Autodesk Inventor part; units mm, degrees
ref_plane "YZ Plane" through (0, 0, 0) normal (1, 0, 0) x (0, 1, 0)
ref_plane "XZ Plane" through (0, 0, 0) normal (0, 1, 0) x (-1, 0, 0)
ref_plane "XY Plane" through (0, 0, 0) normal (0, 0, 1) x (1, 0, 0)
sketch "Sketch1" plane through (0, 0, 0) normal (0, 1, 0) x (-1, 0, 0)
  line L0 (44.45, 203.2) -> (-44.45, 203.2)
  line L1 (-44.45, 203.2) -> (-44.45, -203.2)
  line L2 (-44.45, -203.2) -> (44.45, -203.2)
  line L3 (44.45, -203.2) -> (44.45, 203.2)
  line L4 (44.45, 203.2) -> (-44.45, -203.2) construction
  line L5 (-44.45, 203.2) -> (44.45, -203.2) construction
  line L6 (-44.45, 203.2) -> (-20.955, 203.2)
  line L7 (-20.955, 203.2) -> (-20.955, 88.9) construction
  line L8 (-44.45, 88.9) -> (-44.45, 203.2)
  circle A0 centre (-20.955, 88.9) radius 15.494 construction
  line L9 (44.45, 203.2) -> (44.45, 111.6492)
  line L10 (44.45, 203.2) -> (44.45, 38.1)
  line L11 (44.45, 38.1) -> (22.225, 38.1) construction
  circle A1 centre (22.225, 38.1) radius 12.065 construction
  line L12 (-66.675, 88.9) -> (0, 88.9) construction
  line L13 (0, 88.9) -> (0, 203.2) construction
  line L14 (0, 203.2) -> (-66.675, 203.2)
  line L15 (-66.675, 203.2) -> (-66.675, 88.9) construction
  line L16 (-66.675, 203.2) -> (-66.675, 209.55) construction
  line L17 (-66.675, 209.55) -> (32.5679, 44.312) construction
  circle A2 centre (-20.955, 104.394) radius 1.5
  circle A3 centre (-34.3732, 96.647) radius 1.5
  circle A4 centre (-34.3732, 81.153) radius 1.5
  circle A5 centre (-20.955, 73.406) radius 1.5
  circle A6 centre (-7.5368, 81.153) radius 1.5
  circle A7 centre (-7.5368, 96.647) radius 1.5
  circle A8 centre (-20.955, 88.9) radius 7.112 construction
  circle A9 centre (-28.067, 88.9) radius 5.9944
  line L18 (-20.955, 88.9) -> (-20.955, 152.4) construction
  circle A10 centre (-20.955, 152.4) radius 8.001 construction
  circle A11 centre (-20.955, 152.4) radius 4.0005
  circle A12 centre (-20.955, 160.401) radius 1.85
  line L19 (42.545, 152.4) -> (-20.955, 152.4) construction
  circle A13 centre (-28.956, 152.4) radius 1.85
  line L20 (-20.955, 215.9) -> (-20.955, 152.4) construction
  circle A14 centre (-20.955, 144.399) radius 1.85
  line L21 (-84.455, 152.4) -> (-20.955, 152.4) construction
  circle A15 centre (-12.954, 152.4) radius 1.85
  line L22 (44.45, 0) -> (-44.45, 0) construction
  circle A16 centre (22.225, 38.1) radius 2.9766
  circle A17 centre (22.225, -38.1) radius 2.9766
  circle A18 centre (-33.8743, 119.8397) radius 12.065 construction
  circle A19 centre (-33.8743, 119.8397) radius 2.9766
  circle A20 centre (-20.955, 152.4) radius 50.8 construction
  line L23 (32.5679, 44.312) -> (22.7595, 60.6429) construction
  line L24 (22.7595, 60.6429) -> (17.8553, 68.8083) construction
  line L25 (15.6729, 78.6085) -> (25.4813, 62.2776)
  line L26 (25.4813, 62.2776) -> (20.0377, 59.0081)
  line L27 (20.0377, 59.0081) -> (10.2292, 75.339)
  line L28 (10.2292, 75.339) -> (15.6729, 78.6085)
  line L29 (15.6729, 78.6085) -> (20.0377, 59.0081) construction
  line L30 (25.4813, 62.2776) -> (10.2292, 75.339) construction
  line L31 (-3.944, 111.2702) -> (5.8645, 94.9394)
  line L32 (-9.3876, 108.0008) -> (-3.944, 111.2702)
  line L33 (5.8645, 94.9394) -> (0.4208, 91.6699)
  line L34 (0.4208, 91.6699) -> (-9.3876, 108.0008)
  line L35 (-23.5608, 143.932) -> (-13.7524, 127.6011)
  line L36 (-29.0044, 140.6625) -> (-23.5608, 143.932)
  line L37 (-13.7524, 127.6011) -> (-19.196, 124.3316)
  line L38 (-19.196, 124.3316) -> (-29.0044, 140.6625)
  circle A21 centre (-20.955, -104.394) radius 1.5
  circle A22 centre (-34.3732, -81.153) radius 1.5
  circle A23 centre (-7.5368, -81.153) radius 1.5
  circle A24 centre (-28.067, -88.9) radius 5.9944
  circle A25 centre (-20.955, -152.4) radius 4.0005
  circle A26 centre (-28.956, -152.4) radius 1.85
  circle A27 centre (-12.954, -152.4) radius 1.85
  circle A28 centre (22.225, -38.1) radius 2.9766
  circle A29 centre (-33.8743, -119.8397) radius 2.9766
  circle A30 centre (-29.2932, -53.9743) radius 3.175
  circle A31 centre (-28.067, 88.9) radius 31.75 construction
  line L39 (-28.067, 88.9) -> (-44.45, 88.9) construction
  line L40 (-44.45, 88.9) -> (-44.45, 12.7)
  line L41 (44.45, 203.2) -> (34.925, 203.2)
  line L42 (34.925, 203.2) -> (34.925, 193.675) construction
  line L43 (34.925, 193.675) -> (44.45, 193.675) construction
  line L44 (44.45, 193.675) -> (44.45, 203.2)
  circle A32 centre (34.925, 193.675) radius 3.175
  line L45 (-44.45, 0) -> (-31.75, 0)
  circle A33 centre (-31.75, 0) radius 3.175
  circle A34 centre (34.925, -193.675) radius 3.175
  line L46 (-44.45, 0) -> (-19.455, 0) construction
  line L47 (-16.28, -76.0639) -> (-22.63, -76.0639) construction
  line L48 (-22.63, -76.0639) -> (-22.63, 51.9267) construction
  line L49 (-22.63, 51.9267) -> (-16.28, 51.9267) construction
  line L50 (-16.28, 51.9267) -> (-16.28, -76.0639) construction
  line L51 (-16.28, -63.9953) -> (-22.63, 63.9953) construction
  line L52 (-22.63, -63.9953) -> (-16.28, 63.9953) construction
  line L53 (-16.28, 51.9267) -> (-22.63, -76.0639) construction
  line L54 (-22.63, 51.9267) -> (-16.28, -76.0639) construction
  line L55 (-16.28, -2.5436) -> (-22.63, -2.5436)
  line L56 (-22.63, -2.5436) -> (-22.63, -21.5936)
  line L57 (-22.63, -21.5936) -> (-16.28, -21.5936)
  line L58 (-16.28, -21.5936) -> (-16.28, -2.5436)
  line L59 (-16.28, -2.5436) -> (-22.63, -21.5936) construction
  line L60 (-22.63, -2.5436) -> (-16.28, -21.5936) construction
  line L61 (-16.28, -40.6436) -> (-22.63, -40.6436)
  line L62 (-16.28, -59.6936) -> (-16.28, -40.6436)
  line L63 (-22.63, -40.6436) -> (-22.63, -59.6936)
  line L64 (-22.63, -59.6936) -> (-16.28, -59.6936)
  line L65 (-16.28, 35.5564) -> (-22.63, 35.5564)
  line L66 (-16.28, 16.5064) -> (-16.28, 35.5564)
  line L67 (-22.63, 35.5564) -> (-22.63, 16.5064)
  line L68 (-22.63, 16.5064) -> (-16.28, 16.5064)
  line L69 (-16.28, -2.5436) -> (-22.63, -2.5436)
  line L70 (-16.28, -21.5936) -> (-16.28, -2.5436)
  line L71 (-22.63, -2.5436) -> (-22.63, -21.5936)
  line L72 (-22.63, -21.5936) -> (-16.28, -21.5936)
  line L73 (44.45, -203.2) -> (25.4, -203.2)
  line L74 (25.4, -203.2) -> (25.4, -128.2) construction
  line L75 (25.4, -128.2) -> (44.45, -128.2) construction
  line L76 (44.45, -128.2) -> (44.45, -203.2)
  circle A35 centre (25.4, -128.2) radius 6.35 construction
  circle A36 centre (25.4, -128.2) radius 9.779 construction
  circle A37 centre (15.621, -128.2) radius 1.778
  circle A38 centre (25.4, -128.2) radius 6.35 construction
  circle A39 centre (25.4, -128.2) radius 9.779 construction
  line L77 (100.4, -128.2) -> (25.4, -128.2) construction
  line L78 (25.4, -128.2) -> (25.4, -109.15) construction
  circle A40 centre (25.4, -137.979) radius 1.778
  circle A41 centre (25.4, -128.2) radius 6.35 construction
  circle A42 centre (25.4, -128.2) radius 9.779 construction
  line L79 (25.4, -53.2) -> (25.4, -128.2) construction
  line L80 (25.4, -128.2) -> (6.35, -128.2) construction
  circle A43 centre (35.179, -128.2) radius 1.778
  circle A44 centre (25.4, -128.2) radius 6.35 construction
  circle A45 centre (25.4, -128.2) radius 9.779 construction
  line L81 (-49.6, -128.2) -> (25.4, -128.2) construction
  line L82 (25.4, -128.2) -> (25.4, -147.25) construction
  circle A46 centre (25.4, -118.421) radius 1.778
  point P0 (0, 0)
  point P1 (-19.455, -12.0686)
  dimension "d4" = 30.988
  dimension "d7" = 24.13
  dimension "d16" = 14.224
  dimension "d19" = 16.002
  dimension "d74" = 19.558
  dimension "d0" = 88.9
  dimension "d1" = 406.4
  dimension "d2" = 114.3
  dimension "d3" = 23.495
  dimension "d5" = 165.1
  dimension "d6" = 22.225
  dimension "d10" = 6.35
  dimension "d14" = 360
  dimension "d17" = 11.9888
  dimension "d18" = 63.5
  dimension "d20" = 8.001
  dimension "d21" = 3.7
  dimension "d24" = 360
  dimension "d26" = 5.9531
  dimension "d27" = 24.13
  dimension "d28" = 5.9531
  dimension "d29" = 101.6
  dimension "d32" = 19.05
  dimension "d33" = 9.525
  dimension "d34" = 6.35
  dimension "d37" = 38.1
  dimension "d48" = 63.5
  dimension "d50" = 9.525
  dimension "d51" = 9.525
  dimension "d52" = 6.35
  dimension "d53" = 12.7
  dimension "d54" = 6.35
  dimension "d57" = 6.35
  dimension "d58" = 127.9906
  dimension "d59" = 6.35
  dimension "d60" = 19.05
  dimension "d63" = 38.1
  dimension "d66" = 38.1
  dimension "d71" = 75
  dimension "d72" = 19.05
  dimension "d73" = 12.7
  dimension "d75" = 3.556
  dimension "d78" = 360
extrude "Extrusion6" add sketch "Sketch1" along normal blind 6.35 contours L3 L2 L1 L0 | A2 | A4 | A6 | A12 | A14
properties part number "ChassisOutide10"
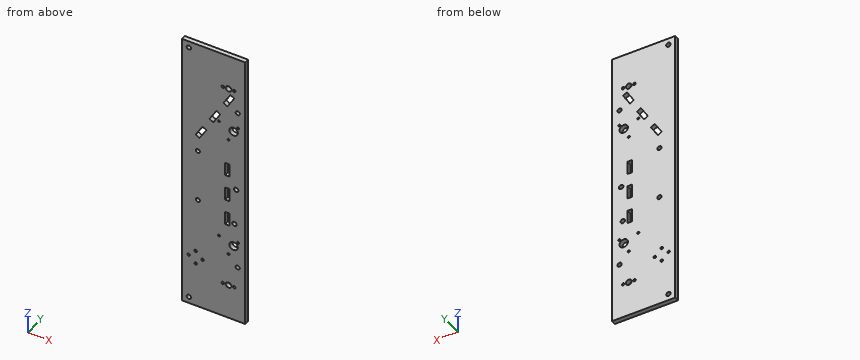
Build history of the part. All positions in model axes, mm. Coordinates: 2 decimals unless noted, no trailing zeros. Order: outer loops, then holes, each group sorted by start corner. A loop starts at its lowest first (then second) coordinate and runs counter-clockwise, first axis right, second up.
Item 1: Drill centre lines: L1, parallel to X at y = 3, z = -128.2; L2, parallel to X at y = 4.75, z = -54; L3, parallel to Z at x = -26, y = 3.25. Where is each one in solid material? Low to high.
Filled in:
L1: x = -44.45 to -36.96, -33.4 to -17.4, -13.84 to 44.45
L2: x = -44.45 to 16.28, 22.63 to 26.12, 32.47 to 44.45
L3: z = -203.2 to -139.65, -136.31 to -120.09, -116.75 to 203.2
Item 2: Drop flat-ended pins along their axis: pin 1 Ø4 at (x, z) = (34.37, -81.15) entering from -Y; pin 2 Ø3 at (x, z) = (28.956, 152.4) entering from +Y. Give the stop position or say it passes through.
Filled in:
pin 1: stops at y = 0
pin 2: passes through
Item 3: Saw through at B-B on y = 1. State how many separate pieces and enclosed holes the cut face has, then the cut area to 3 significant figures.
Filled in:
separate pieces: 1
enclosed holes: 32
area: 34,700 mm2
Item 4: Saw through at A-A on z = -88.9. List the corners of the cut face in (x, y).
Filled in:
outline: (-44.45, 0) - (22.07, 0) - (22.07, 6.35) - (-44.45, 6.35) - close; (34.06, 0) - (44.45, 0) - (44.45, 6.35) - (34.06, 6.35) - close
Item 5: Saw through at C-C on z = 133. List the corners of the cut face in (x, y) (3 decimals).
Filled in:
outline: (-44.45, 0) - (16.995, 0) - (16.995, 6.35) - (-44.45, 6.35) - close; (24.402, 0) - (44.45, 0) - (44.45, 6.35) - (24.402, 6.35) - close
